Part model, mm, in its own coordinate system. Face numbers are marked on the shaded views. A direction names the side the tool comes from. Round coordinates to 2 decimals unless told otherwise and drop trailing zeros. Loops run counter-clockwise (first coordinate to the right, second up) from the corner with the lowest first, then second, coordinate; pieces in that order, holes last. Notation, with made-up numbers: (41.25, -15) -> (79.25, -15) arc R9 cw to (79.25, -6) -> close; hole circle Ø4 at (-22.75, 5). An arc over 180 degrees is marked (long way). Use a Markdown table: item, result. Add a question column.
Item 1: Two-plate mould, pull along Z, no slides. Class the marked faces 1, 2 and 3: pulls with the +Z half, pulls with the -Z half, needs draft (parallel to the pull), parting line crosses it, or undercut.
Item 2: Probe line 1 (Z direction, x = 0.15, y = 0); line 2 (Z direction, x = -0.45, y = 0); line 3 (Y direction, x = 12.5, z = -1.5). List the from-to ranges inside material, lowest first. Write a range as [from, to].
Item 3: Which spindle directions (+Z, -Z, +X, -X, +Y, -Y) get a long thin tool onto all of the face, cutting with end or side? Do the marked faces 4, 5 and 6. Say none if no direction does.
Item 4: Flat gauge pins, fed straight in: pin 1 (5 mm diameter, centred on y = -3, z = -2.5, fed in from +X); pin 2 (3 mm diameter, centred on x = 10, y = -2, fed in from +Z); pin 3 (2 mm diameter, centred on x = 2.5, y = -0.5, fed in from +Z); pin 4 (1.5 mm diameter, centred on y = 0, z = 0, fed in from -X). Where does each tip first touch, or does it go through?
Item 5: Cut at A-A, the plane x = 6.25. List the corners of the cut face in (y, z).
Autodesk Inventor part; units mm, degrees
ref_plane "Work Plane1" through (8, 0, 0) normal (0, 0.5, 0.866) x (1, 0, 0)
ref_plane "YZ Plane" through (0, 0, 0) normal (1, 0, 0) x (0, 1, 0)
ref_plane "XZ Plane" through (0, 0, 0) normal (0, 1, 0) x (-1, 0, 0)
sketch "Sketch1" plane through (0, 0, 0) normal (0, 0, 1) x (1, 0, 0)
  line L0 (1.2217, 0) -> (16, 0)
  line L1 (16, 0) -> (16, 2.5)
  line L2 (16, 2.5) -> (0, 2.5)
  line L3 (0, 2.5) -> (0, 4.25)
  line L4 (0, 4.25) -> (-3.5, 4.25)
  line L5 (-3.5, 4.25) -> (-3.5, 2.3094)
  line L6 (-3.5, 2.3094) -> (-1.5, 2.3094)
  line L7 (-1.5, 2.3094) -> (-0.8884, 1.25)
  line L8 (-7.4, 0) -> (19.9, 0)
  line L9 (0, -0.85) -> (0, 5.1)
  line L10 (-0.8884, 1.25) -> (0.5, 1.25)
  line L11 (0.5, 1.25) -> (1.2217, 0)
  line L12 (-3.5, 2.3094) -> (-3.5, 0) construction
  line L13 (-3.5, 3.75) -> (-3, 4.25)
  dimension "d0" = 3.5
  dimension "d1" = 2
  dimension "d2" = 60
  dimension "d3" = 5
  dimension "d4" = 4.6188
  dimension "d5" = 8.5
  dimension "d15" = 4
  dimension "d16" = 2.5
  dimension "d17" = 16
  dimension "d32" = 45
  dimension "d33" = 0.5
revolve "Body" add sketch "Sketch1" angle 360 about axis through (1.2217, 0, 0) along (1, 0, 0) contours L11 L10 L9 L2 L1 L0 | L10 L7 L6 L5 L13 L4 L3 L9 | L13 L5 L4
revolve "Chamfer2" cut sketch "Sketch1" angle 360 about axis through (-10, 0, 0) along (1, 0, 0) contours L13 L5 L4
sketch "Sketch2" plane through (-3.5, 0, 0) normal (-1, 0, 0) x (0, 0, 1)
  circle A0 centre (0, 0) radius 2.3094
  line L0 (0, -5.95) -> (0, 5.95)
  line L1 (-5.95, 0) -> (5.95, 0)
  line L2 (2.3094, 0) -> (1.1547, -2)
  line L3 (1.1547, -2) -> (-1.1547, -2)
  line L4 (-1.1547, -2) -> (-2.3094, 0)
  line L5 (-2.3094, 0) -> (-1.1547, 2)
  line L6 (-1.1547, 2) -> (1.1547, 2)
  line L7 (1.1547, 2) -> (2.3094, 0)
extrude "Slot" add sketch "Sketch2" against normal up to next contours L7 A0 | A0 L2 | L6 L0 A0 | A0 L0 L3 | L0 L6 A0 | A0 L3 L0 | L4 A0 | A0 L5
thread "Thread"
chamfer "Chamfer1" distance 0.4908 distance2 0.4908 1 edges at (16, -2.5, 0) measured on face at (16, -1.1374, -1.1324)
ref_plane "Work Plane1" through (8, 0, 0) normal (0, 0.5, 0.866) x (1, 0, 0)
equation "\"d0\" = KOH"
equation "\"d1\" = INTI"
equation "\"d3\" = GD"
equation "\"d4\" = 1.1547 * SW"
equation "\"d5\" = KOD"
equation "\"d15\" = INFT"
equation "\"d16\" = SDT"
equation "\"d17\" = NLG"
equation "\"d33\" = Cham"
equation "\"d7\" = GEL"
equation "\"d9\" = -0.5 * SPD + 0.5 * GD"
equation "\"d12\" = GUL"
equation "\"GD\" = NND"
equation "\"NLG\" = 16"
equation "\"GEL\" = 11.8"
equation "\"KOD\" = 8.5"
equation "\"KOH\" = 3.5"
equation "\"GUL\" = 0.61345 * PTC"
equation "\"SW\" = 4"
equation "\"INTI\" = 2"
equation "\"SPD\" = NND - 1.2269 * PTC"
equation "\"SDT\" = 2.5"
equation "\"INFT\" = 4"
equation "\"Cham\" = 0.5"
equation "\"TOA\" = 30deg"
equation "\"GD1\" = THREADDIA - 1.2269 * PTC"
equation "\"THREADDIA\" = 5"
equation "\"BDM\" = NND"
equation "\"FAWI\" = 45deg"
equation "\"RR\" = 0.1 * NND"
equation "\"PTC\" = 0.8"
equation "\"NND\" = 5"
equation "\"FAWI1\" = 45deg"
equation "\"GAL\" = 0.61345 * PTC"
equation "\"E0\" = 1.155 * SW"
properties part number "DIN 6912 - M5 x 16" material "Steel, Mild"
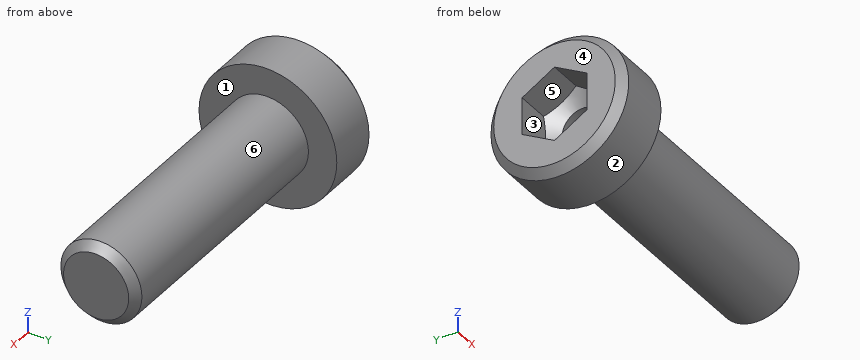
A:
| question | item | result |
|---|---|---|
| 1 | face 1 | needs draft |
| 1 | face 2 | parting line crosses it |
| 1 | face 3 | undercut |
| 2 | line 1 | z = [-2.5, -1.25], [1.25, 2.5] |
| 2 | line 2 | z = [-4.25, -1.25], [1.25, 4.25] |
| 2 | line 3 | y = [-2, 2] |
| 3 | face 4 | +Z, -Z, -X, +Y, -Y |
| 3 | face 5 | -X |
| 3 | face 6 | +X |
| 4 | pin 1 | stops at x = 16 |
| 4 | pin 2 | stops at z = 2.45 |
| 4 | pin 3 | stops at z = 2.5 |
| 4 | pin 4 | stops at x = 0.79 |
| 5 | outline | circle Ø5 at (0, 0) |
